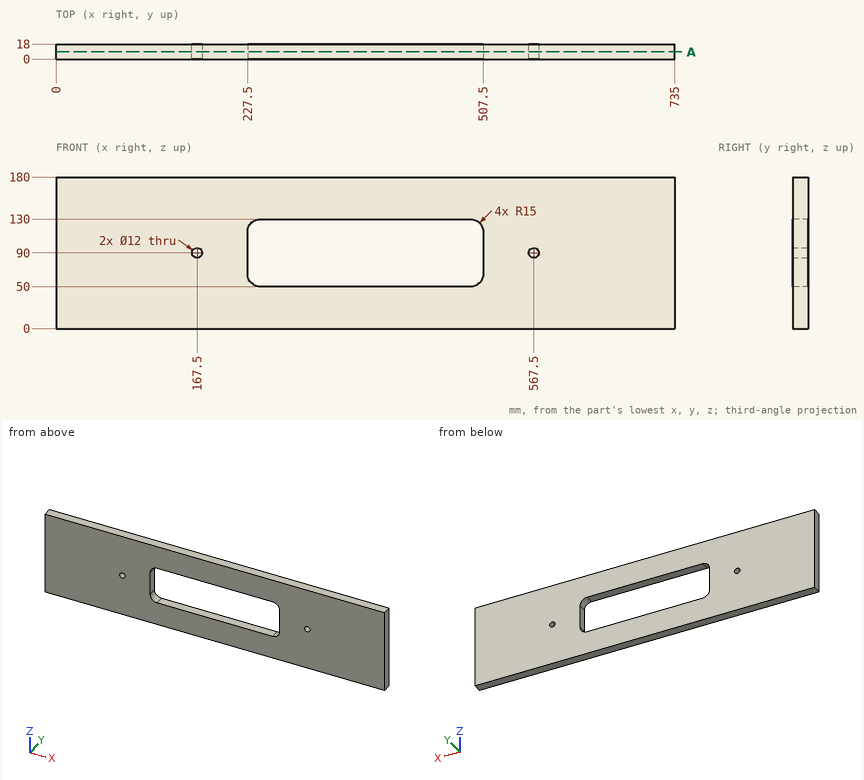
Drawing for the job (mm, zero at the part's lowest x, y, z). Round coordinates to 2 decimals unless told otherwise and drop trailing zeros. Write each loop counter-clockwise with the first axis right and the second up, starting at its lowest first coordinate (ties: lowest second). Pieces come first, ordered by that corner, then holes. Notation, with made-up numbers: (13, -34.5) - (50, -34.5) arc R18 ccw to (50, -13.5) - close; hole circle Ø6 at (-37.75, 13.5). An arc over 180 degrees is marked (long way). Return JSON: item names as keys, results as strings. Group by question number.
Item 1: Probe probe 1 along X at (y, z) = (11, 90); probe 2 along Z at (x, y) = (328, 13); probe 3 along Z at (x, y) = (567.5, 10.25). List the from-to ranges inside material, lowest first.
Item 2: Band-saw the part on A-A on y = 8.5. List the corners of the cut face in (x, z).
Item 3: Flat gauge pins, fed straight in: pin 1 Ø9 at (x, y) = (316.5, 12) entering from -Z; pin 2 Ø7 at (x, z) = (167.5, 90) entering from +Y. Where does each tip first touch, or does it go through?
Resolved:
{
 "1": {"probe 1": "x = 0 to 161.5, 173.5 to 227.5, 507.5 to 561.5, 573.5 to 735", "probe 2": "z = 0 to 50, 130 to 180", "probe 3": "z = 0 to 84, 96 to 180"},
 "2": {"outline": "(0, 0) - (735, 0) - (735, 180) - (0, 180) - close; hole circle Ø12 at (167.5, 90); hole (227.5, 65) arc R15 ccw to (242.5, 50) - (492.5, 50) arc R15 ccw to (507.5, 65) - (507.5, 115) arc R15 ccw to (492.5, 130) - (242.5, 130) arc R15 ccw to (227.5, 115) - close; hole circle Ø12 at (567.5, 90)"},
 "3": {"pin 1": "stops at z = 0", "pin 2": "passes through"}
}
